Part model, mm, in its own coordinate system. A direction names the side the tool comes from. Round coordinates to 2 decimals unless told otherwise and drop trailing zeros. Write each loop counter-clockwise with the first axis right and the second up, starting at its lowest first coordinate (ties: lowest second). Pieces come first, ordered by that corner, then holes.
```python
from build123d import *

# Parameters (mm, degrees)
SKETCH1_R           = 3.000854516
SKETCH1_W           = 5.001424193
SKETCH1_H           = 20.005696775
SKETCH1_W_2         = 20.005696776
SKETCH1_H_2         = 5.001424194
SKETCH1_W_3         = 20.005696775
SKETCH1_W_4         = 5.001424194
BOSS_EXTRUDE1_DEPTH = 5


with BuildPart() as part:
    # Sketch1 → Boss-Extrude1 (new body)
    with BuildSketch(Plane(origin=(0, 0, 0), x_dir=(0, 0, -1), z_dir=(1, 0, 0))):
        with BuildLine():
            Line((-105.391894776, -37.510681454), (44.616650387, -37.510681454))
            Line((44.616650387, -37.510681454), (44.616650387, 17.510681454))
            ThreePointArc((44.616650387, 17.510681454), (38.758786011, 31.652817078), (24.616650387, 37.510681454))
            Line((24.616650387, 37.510681454), (-105.391894776, 37.510681454))
            Line((-105.391894776, 37.510681454), (-105.391894776, -37.510681454))
        make_face()
        with Locations((29.612377806, 22.506408872)):
            Circle(SKETCH1_R, mode=Mode.SUBTRACT)
        with Locations(Location((-90.387622194, 22.506408872, 0), (0, 0, 180))):
            Circle(SKETCH1_R, mode=Mode.SUBTRACT)
        with Locations((2.10454474, -12.503560485)):
            Rectangle(SKETCH1_W, SKETCH1_H, mode=Mode.SUBTRACT)
        with Locations((-5.791359719, 29.352456285)):
            Rectangle(SKETCH1_W_2, SKETCH1_H_2, mode=Mode.SUBTRACT)
        with Locations((-54.98388467, 29.352456285)):
            Rectangle(SKETCH1_W_3, SKETCH1_H_2, mode=Mode.SUBTRACT)
        with Locations((-62.879789128, -12.503560485)):
            Rectangle(SKETCH1_W_4, SKETCH1_H, mode=Mode.SUBTRACT)
    extrude(amount=BOSS_EXTRUDE1_DEPTH)


solid = part.part
```
Q1. Mould opens along Y. For faces 1 (the flat face through (2, -10, -44.617)), 2 (the flat face through (2, 37.511, 39)), 3 (the flat face through (2, -13, -4.605)) say: +Y half, -Y half, draft (parallel to the pull), parting line (faces both ways), or undercut.
Values follow:
face 1: draft
face 2: +Y half
face 3: undercut
Q2. Cut at C-C on x = 0.8. Write the cut outline in (y, z).
Values follow:
outline: (-37.51, -44.62) - (17.51, -44.62) arc R20 ccw to (37.51, -24.62) - (37.51, 105.39) - (-37.51, 105.39) - close; hole (-22.51, -4.61) - (-2.5, -4.61) - (-2.5, 0.4) - (-22.51, 0.4) - close; hole (-22.51, 60.38) - (-2.5, 60.38) - (-2.5, 65.38) - (-22.51, 65.38) - close; hole circle Ø6 at (22.51, -29.61); hole circle Ø6 at (22.51, 90.39); hole (26.85, -4.21) - (31.85, -4.21) - (31.85, 15.79) - (26.85, 15.79) - close; hole (26.85, 44.98) - (31.85, 44.98) - (31.85, 64.99) - (26.85, 64.99) - close
Q3. Cut at A-A on z = 13. Write the cut outline in (x, y), plus the area to 3 significant figures.
Values follow:
outline: (0, -37.51) - (5, -37.51) - (5, 26.85) - (0, 26.85) - close; (0, 31.85) - (5, 31.85) - (5, 37.51) - (0, 37.51) - close
area: 350 mm2
Q4. Cut at B-B on y = -6. Write the cut outline in (x, z), plus the area to 3 significant figures.
Values follow:
outline: (0, -44.62) - (5, -44.62) - (5, -4.61) - (0, -4.61) - close; (0, 0.4) - (5, 0.4) - (5, 60.38) - (0, 60.38) - close; (0, 65.38) - (5, 65.38) - (5, 105.39) - (0, 105.39) - close
area: 700 mm2
Q5. Which spindle directions (+Z, -Z, +X, -X, +Y, -Y) get a long thin tool onto all of the face, cutting with end or side? Do faces 4 (the flat face through (0, 1, 31)), 5 (the flat face through (2, 31.853, 6)). Say none if no direction does.
Values follow:
face 4: +Z, -Z, -X, +Y, -Y
face 5: +X, -X
Q6. Wall check: L1, parallel to Z at x = 4.45, y = -16.5; L2, parallel to Y at x = 2.15, z = 5; L3, parallel to Z at x = 0.75, y = 28.5. Give the ranges that are in metal, low to high.
Values follow:
L1: z = -44.62 to -4.61, 0.4 to 60.38, 65.38 to 105.39
L2: y = -37.51 to 26.85, 31.85 to 37.51
L3: z = -41.33 to -4.21, 15.79 to 44.98, 64.99 to 105.39
Q7. Cut at D-D on z = -29. Write the cut outline in (x, y).
Values follow:
outline: (0, -37.51) - (5, -37.51) - (5, 19.57) - (0, 19.57) - close; (0, 25.44) - (5, 25.44) - (5, 37.02) - (0, 37.02) - close
Q8. Drop flat-ended pins along their axis: pin 1 (1 mm diameter, centred on y = -8.5, z = 85, fed in from -X); pin 2 (5 mm diameter, centred on y = 22.51, z = 90.39, fed in from -X). Give the stop position or say it passes through.
Values follow:
pin 1: stops at x = 0
pin 2: passes through
